from build123d import *

# Parameters (mm, degrees)
F1_DEPTH = 127
F0_R     = 50.8
F2_DEPTH = 50.8
F3_DEPTH = 25.4


with BuildPart() as f1:
    # F0 (on Front) → F1 (new body)
    with BuildSketch(Plane.XZ):
        Polygon((255.951391, 57.862211), (255.951391, 121.362211), (0, 121.362211), (0, 57.862211), (65.451391, 57.862211), (27.351391, 95.962211), (230.551391, 95.962211), (192.451391, 57.862211), align=None)
    extrude(amount=F1_DEPTH)

    # F0 (on Front) → F2 (join)
    with BuildSketch(Plane.XZ):
        Polygon((255.951391, 57.862211), (255.951391, 121.362211), (0, 121.362211), (0, 57.862211), (65.451391, 57.862211), (27.351391, 95.962211), (230.551391, 95.962211), (192.451391, 57.862211), align=None)
        with BuildLine():
            ThreePointArc((216.875695, 215.35869), (215.571015, 230.533337), (211.69527, 245.262584))
            ThreePointArc((211.69527, 245.262584), (127.975695, 304.25869), (44.256121, 245.262584))
            ThreePointArc((44.256121, 245.262584), (112.801048, 127.76337), (216.875695, 215.35869))
        make_face()
        with Locations((127.975695, 215.35869)):
            Circle(F0_R, mode=Mode.SUBTRACT)
        with BuildLine():
            Line((0, 121.362211), (255.951391, 121.362211))
            Line((255.951391, 121.362211), (211.69527, 245.262584))
            ThreePointArc((211.69527, 245.262584), (215.571015, 230.533337), (216.875695, 215.35869))
            ThreePointArc((216.875695, 215.35869), (112.801048, 127.76337), (44.256121, 245.262584))
            Line((44.256121, 245.262584), (0, 121.362211))
        make_face()
    extrude(amount=-F2_DEPTH)

    # F0 (on Front) → F3 (join)
    with BuildSketch(Plane.XZ):
        with BuildLine():
            ThreePointArc((216.875695, 215.35869), (215.571015, 230.533337), (211.69527, 245.262584))
            ThreePointArc((211.69527, 245.262584), (127.975695, 304.25869), (44.256121, 245.262584))
            ThreePointArc((44.256121, 245.262584), (112.801048, 127.76337), (216.875695, 215.35869))
        make_face()
        with Locations((127.975695, 215.35869)):
            Circle(F0_R, mode=Mode.SUBTRACT)
    extrude(amount=F3_DEPTH)


solid = f1.part
The model under review builds one solid part; all positions refer to its coordinate system, in mm. A direction names the side the tool comes from. Coordinates: 2 decimals unless noted, no trailing zeros. Loops run counter-clockwise (first coordinate to the right, second up) from the corner with the lowest first, then second, coordinate; pieces in that order, holes last.
(1) Consider section A-A, the plane y = 27. Give the boundary of the cut face in (x, z).
Determined:
outline: (0, 57.86) - (65.45, 57.86) - (27.35, 95.96) - (230.55, 95.96) - (192.45, 57.86) - (255.95, 57.86) - (255.95, 121.36) - (211.7, 245.26) arc R88.9 ccw to (44.26, 245.26) - (0, 121.36) - close; hole circle Ø101.6 at (127.98, 215.36)
(2) Wall thickness on L1, parallel to Z at x = 160, y = -1.5; L2, parallel to Y at x = 205, z = 131.5; L3, parallel to X at y = 5, z = 89: over which ranges is each line inside the solid? List them lowest first.
Determined:
L1: z = 95.96 to 121.36, 132.43 to 175.92, 254.79 to 298.29
L2: y = 0 to 50.8
L3: x = 0 to 34.31, 223.59 to 255.95
(3) Insertion check: P1, Ø6, axis at y = -22.5, z = 271.5, coming from the -X side; P2, Ø5, axis at y = -18, z = 136, coming from the +X side; P3, Ø5, axis at y = 33, z = 206.5, coming from the -X side. Each pin has a flat end and moves straight along its axis. Give the tip position at first contact, or say it passes through.
Determined:
P1: stops at x = 56.71
P2: stops at x = 172.65
P3: stops at x = 29.52
(4) Consider section D-D, the plane y = -103. Give the boundary of the cut face in (x, z).
Determined:
outline: (0, 57.86) - (65.45, 57.86) - (27.35, 95.96) - (230.55, 95.96) - (192.45, 57.86) - (255.95, 57.86) - (255.95, 121.36) - (0, 121.36) - close
(5) Consider section C-C, the plane z = 226. Give the boundary of the cut face in (x, y).
Determined:
outline: (37.38, 0) - (39.71, 0) - (39.71, -25.4) - (78.3, -25.4) - (78.3, 50.8) - (37.38, 50.8) - close; (177.65, -25.4) - (216.24, -25.4) - (216.24, 0) - (218.58, 0) - (218.58, 50.8) - (177.65, 50.8) - close
(6) Tool access review of faces 1 (the flat face through (127, 0, 124)), 2 (the cylindrical face through (215.607, -12.522, 230.323)), 3 (the flat face through (166, -25.4, 177)), 4 (the flat face through (128, -39, 95.962)), 5 (the flat face through (130, -63, 121.362)): name each direction out of +Z, -Z, +X, -X, +Y, -Y from which nothing blocks a thin tool from reaching the whole face with its end or side.
Determined:
face 1: -Y
face 2: +Z, +X, -Y
face 3: +Z, +X, -X, -Y
face 4: +Y, -Y
face 5: +X, -X, -Y
(7) Consider section B-B, the plane x = 116.5. Give the boundary of the cut face in (y, z).
Determined:
outline: (-127, 95.96) - (50.8, 95.96) - (50.8, 165.87) - (-25.4, 165.87) - (-25.4, 127.2) - (0, 127.2) - (0, 121.36) - (-127, 121.36) - close; (-25.4, 264.85) - (50.8, 264.85) - (50.8, 303.51) - (-25.4, 303.51) - close
(8) Draft analysis for pull direction X (two halves, no side actions). For faces 6 (the flat face through (22.44, 25.04, 184.18)), 7 (the flat face through (255.951, -39, 89)), 8 (the flat face through (211.77, -39.34, 77.18)), 9 (the flat face through (46.668, -39.345, 76.646)), state which applies: +X half, -X half, draft (parallel to the pull), parting line (faces both ways), or undercut.
Determined:
face 6: -X half
face 7: +X half
face 8: undercut
face 9: undercut
